The model under review builds one solid part; all positions refer to its coordinate system, in mm. Coordinates: 2 decimals unless noted, no trailing zeros. Loops run counter-clockwise (first coordinate to the right, second up) from the corner with the lowest first, then second, coordinate; pieces in that order, holes last. Notation, with made-up numbers: M -15,77 L 27,77 A29 cw 27,97 Z; hole C 41.5,86.5 d3. An arc over 180 degrees is marked long. One line per item, written item: value.
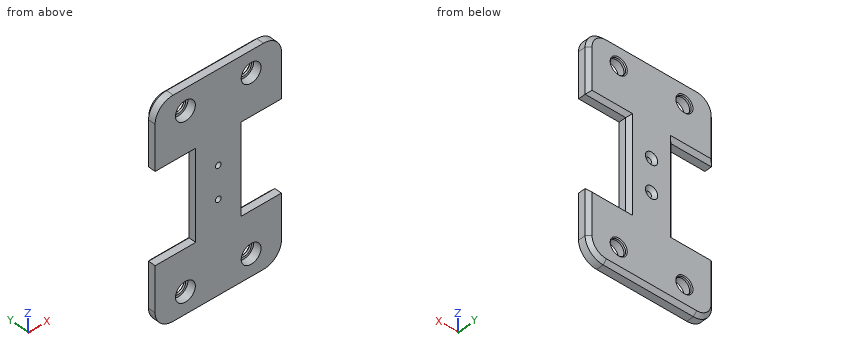
```python
from build123d import *

# Parameters (mm, degrees)
ESQUISSE2_R             = 4.25
ESQUISSE2_R_2           = 1.6
BOSS_EXTRU_1_DEPTH      = 6
CONG_1_R                = 10
CHANFREIN1_SIZE         = 1.8
CHANFREIN2_SIZE         = 2
ESQUISSE3_R             = 5.5
ENL_V_MAT_EXTRU_1_DEPTH = 4.5
CHANFREIN3_SIZE         = 0.5


with BuildPart() as part:
    # Esquisse2 → Boss.-Extru.1 (new body)
    with BuildSketch(Plane(origin=(0, 0, 0), x_dir=(1, 0, 0), z_dir=(0, 1, 0))):
        Polygon((-12.5, -25), (-12.5, 25), (-35, 25), (-35, 60), (35, 60), (35, 25), (12.5, 25), (12.5, -25), (35, -25), (35, -60), (-35, -60), (-35, -25), align=None)
        with Locations((-18.2, 48)):
            Circle(ESQUISSE2_R, mode=Mode.SUBTRACT)
        with Locations((18.2, 48)):
            Circle(ESQUISSE2_R, mode=Mode.SUBTRACT)
        with Locations((18.2, -48)):
            Circle(ESQUISSE2_R, mode=Mode.SUBTRACT)
        with Locations((-18.2, -48)):
            Circle(ESQUISSE2_R, mode=Mode.SUBTRACT)
        with Locations((0, 9)):
            Circle(ESQUISSE2_R_2, mode=Mode.SUBTRACT)
        with Locations((0, -9)):
            Circle(ESQUISSE2_R_2, mode=Mode.SUBTRACT)
    extrude(amount=BOSS_EXTRU_1_DEPTH)

    # Congé1
    cong_1_edges = [part.edges().sort_by_distance(p)[0] for p in [
        (-35, 3, -60),
        (35, 3, -60),
        (35, 3, 60),
        (-35, 3, 60),
    ]]
    fillet(cong_1_edges, radius=CONG_1_R)

    # Chanfrein1
    chanfrein1_edges = [part.edges().sort_by_distance(p)[0] for p in [
        (-1.6, 6, -9),
        (-1.6, 6, 9),
    ]]
    chamfer(chanfrein1_edges, length=CHANFREIN1_SIZE)

    # Chanfrein2
    chanfrein2_edges = [part.edges().sort_by_distance(p)[0] for p in [
        (-23.75, 6, 25),
        (-35, 6, 37.5),
        (23.75, 6, 25),
        (12.5, 6, 0),
        (23.75, 6, -25),
        (35, 6, -37.5),
        (-23.75, 6, -25),
        (0, 6, 60),
        (35, 6, 37.5),
        (0, 6, -60),
        (-35, 6, -37.5),
        (-32.071067812, 6, -57.071067812),
        (32.071067812, 6, -57.071067812),
        (32.071067812, 6, 57.071067812),
        (-32.071067812, 6, 57.071067812),
        (-12.5, 6, 0),
    ]]
    chamfer(chanfrein2_edges, length=CHANFREIN2_SIZE)

    # Esquisse3 → Enlèv. mat.-Extru.1 (cut)
    with BuildSketch(Plane.XZ):
        with Locations((-18.2, 48)):
            Circle(ESQUISSE3_R)
        with Locations((18.2, 48)):
            Circle(ESQUISSE3_R)
        with Locations((18.2, -48)):
            Circle(ESQUISSE3_R)
        with Locations((-18.2, -48)):
            Circle(ESQUISSE3_R)
    extrude(amount=-ENL_V_MAT_EXTRU_1_DEPTH, mode=Mode.SUBTRACT)

    # Chanfrein3
    chanfrein3_edges = [part.edges().sort_by_distance(p)[0] for p in [
        (-22.45, 6, -48),
        (13.95, 6, -48),
        (13.95, 6, 48),
        (-22.45, 6, 48),
    ]]
    chamfer(chanfrein3_edges, length=CHANFREIN3_SIZE)


solid = part.part
```
(1) Add section A-A on y = 2. State the section outline as (x, z) points.
Checks:
outline: M -35,-50 A10 ccw -25,-60 L 25,-60 A10 ccw 35,-50 L 35,-25 L 12.5,-25 L 12.5,25 L 35,25 L 35,50 A10 ccw 25,60 L -25,60 A10 ccw -35,50 L -35,25 L -12.5,25 L -12.5,-25 L -35,-25 Z; hole C -18.2,-48 d11; hole C -18.2,48 d11; hole C 0,-9 d3.2; hole C 0,9 d3.2; hole C 18.2,-48 d11; hole C 18.2,48 d11
(2) To check wall thickness, follow L1, parallel to Z at x = -18.2, y = 2.55; L2, parallel to Z at x = 0, y = 1.15; L3, parallel to X at y = 4.9, z = -48. State the ranges of each line that lie inside material, in increasing order. Write a range as [from, to].
Checks:
L1: [-60, -53.5], [-42.5, -25], [25, 42.5], [53.5, 60]
L2: [-60, -10.6], [-7.4, 7.4], [10.6, 60]
L3: [-34.1, -22.45], [-13.95, 13.95], [22.45, 34.1]
(3) Insertion check: pin 1 Ø2 at (y, z) = (1.5, 11.5) entering from -X; pin 2 Ø5.5 at (x, z) = (20, -47.5) entering from -Y; pin 3 Ø1 at (x, y) = (26, 4) entering from +Z. Each pin has a flat end and moves straight along its axis. Give the tip position at first contact, or say it passes through.
Checks:
pin 1: x = -12.5
pin 2: y = 4.5
pin 3: z = 59.99
(4) Add section B-B on z = 48. State the section outline as (x, y) points.
Checks:
outline: M -35,0 L -23.7,0 L -23.7,4.5 L -22.45,4.5 L -22.45,5.5 L -22.95,6 L -33,6 L -35,4 Z; M -13.95,4.5 L -12.7,4.5 L -12.7,0 L 12.7,0 L 12.7,4.5 L 13.95,4.5 L 13.95,5.5 L 13.45,6 L -13.45,6 L -13.95,5.5 Z; M 22.45,4.5 L 23.7,4.5 L 23.7,0 L 35,0 L 35,4 L 33,6 L 22.95,6 L 22.45,5.5 Z
(5) Add section D-D on x = -18.2. State how many separate pieces and enclosed holes the cut face has, then the cut area to 3 significant figures.
Checks:
separate pieces: 4
enclosed holes: 0
area: 287 mm^2
(6) Add section C-C on x = 0. State the section outline as (y, z) points, then the cut area to 3 significant figures.
Checks:
outline: M 0,-60 L 4,-60 L 6,-58 L 6,-12.4 L 4.2,-10.6 L 0,-10.6 Z; M 0,-7.4 L 4.2,-7.4 L 6,-5.6 L 6,5.6 L 4.2,7.4 L 0,7.4 Z; M 0,10.6 L 4.2,10.6 L 6,12.4 L 6,58 L 4,60 L 0,60 Z
area: 671 mm^2
